Can you work these out from the model? Positions are in its coordinate system, mm. Face numbers are marked on the shaded views. A direction names the side the tool comes from. Give positions to 0.01 mm unless a question says otherwise; leave off trailing zeros. Loops run counter-clockwise (first coordinate to the right, second up) from the corner with the lowest first, then second, coordinate; pieces in that order, holes last.
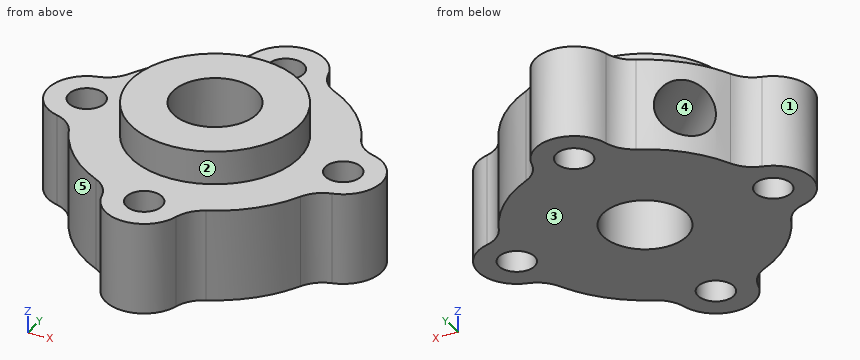
from build123d import *

# Parameters (mm, degrees)
BOSS_EXTRUDE2_DEPTH   = 6.985
FILLET3_R             = 2.54
SKETCH2_R             = 6.35
BOSS_EXTRUDE3_DEPTH   = 2.54
SKETCH3_R             = 3.175
CUT_EXTRUDE1_DEPTH    = 9.525
F_6_32_TAPPED_HOLE1_D = 2.7051
SKETCH12_R            = 2.159
CUT_EXTRUDE4_DEPTH    = 9.906


with BuildPart() as part:
    # Sketch1 → Boss-Extrude2 (new body)
    with BuildSketch(Plane.XY):
        with BuildLine():
            ThreePointArc((-21.795940027, 25.899130336), (-25.822498312, 23.471180796), (-28.250447852, 19.444622511))
            ThreePointArc((-28.250447852, 19.444622511), (-31.607701099, 16.556383583), (-28.250447852, 13.668144655))
            ThreePointArc((-28.250447852, 13.668144655), (-25.822498312, 9.64158637), (-21.795940027, 7.21363683))
            ThreePointArc((-21.795940027, 7.21363683), (-18.907701099, 3.856383583), (-16.019462171, 7.21363683))
            ThreePointArc((-16.019462171, 7.21363683), (-11.992903886, 9.64158637), (-9.564954346, 13.668144655))
            ThreePointArc((-9.564954346, 13.668144655), (-6.207701099, 16.556383583), (-9.564954346, 19.444622511))
            ThreePointArc((-9.564954346, 19.444622511), (-11.992903886, 23.471180796), (-16.019462171, 25.899130336))
            ThreePointArc((-16.019462171, 25.899130336), (-18.907701099, 29.256383583), (-21.795940027, 25.899130336))
        make_face()
    extrude(amount=BOSS_EXTRUDE2_DEPTH)

    # Fillet3
    fillet3_edges = [part.edges().sort_by_distance(p)[0] for p in [
        (-16.019462171, 7.21363683, 3.4925),
        (-21.795940027, 7.21363683, 3.4925),
        (-28.250447852, 13.668144655, 3.4925),
        (-28.250447852, 19.444622511, 3.4925),
        (-21.795940027, 25.899130336, 3.4925),
        (-16.019462171, 25.899130336, 3.4925),
        (-9.564954346, 19.444622511, 3.4925),
        (-9.564954346, 13.668144655, 3.4925),
    ]]
    fillet(fillet3_edges, radius=FILLET3_R)

    # Sketch2 → Boss-Extrude3 (add)
    with BuildSketch(Plane.XY.offset(6.985)):
        with Locations((-18.907701099, 16.556383583)):
            Circle(SKETCH2_R)
    extrude(amount=BOSS_EXTRUDE3_DEPTH)

    # Sketch3 → Cut-Extrude1 (cut)
    with BuildSketch(Plane.XY.offset(9.525)):
        with Locations((-18.907701099, 16.556383583)):
            Circle(SKETCH3_R)
    extrude(amount=-CUT_EXTRUDE1_DEPTH, mode=Mode.SUBTRACT)

    # #6-32 Tapped Hole1 (through all)
    with Locations(Plane(origin=(0, 0, 0), x_dir=(-1, 0, 0), z_dir=(0, 0, -1))):
        with Locations((18.907701099, 26.335383583), (28.686701099, 16.556383583), (18.907701099, 6.777383583), (9.128701099, 16.556383583)):
            Hole(F_6_32_TAPPED_HOLE1_D / 2)

    # Sketch12 → Cut-Extrude4 (cut)
    with BuildSketch(Plane(origin=(-24.434266922, 24.837342139, 0), x_dir=(0.712867541, 0.701298701, 0), z_dir=(-0.701298701, 0.712867541, 0))):
        with Locations((-1.965596828, -3.45963024)):
            Circle(SKETCH12_R)
    extrude(amount=-CUT_EXTRUDE4_DEPTH, mode=Mode.SUBTRACT)


solid = part.part
(1) Please list where these lines run through material, in increasing order: probe 1 along X at (y, z) = (16.5, 9.25); probe 2 along Z at (x, y) = (-24.25, 23) (3 decimals); probe 3 along Z at (x, y) = (-12.75, 10.75) (3 decimals).
Returned:
probe 1: x = -25.26 to -22.08, -15.73 to -12.56
probe 2: z = 0 to 1.458, 5.462 to 6.985
probe 3: z = 0 to 6.985
(2) Will these pins go through, and if not, where does the flat tip stop? P1, Ø3, axis at x = -21.5, z = 6, coming from the -Y side; P2, Ø4, axis at y = 18.5, z = 8.5, coming from the -X side; P3, Ø4.5, axis at x = -18.91, y = 6.78, coming from the +Z side (3 decimals).
Returned:
P1: stops at y = 4.07
P2: stops at x = -31.54
P3: stops at z = 6.985
(3) Which directions (+Z, -Z, +X, -X, +Y, -Y) give clear straight access to the entire face, cutting with the end or side of a thin tool? Please do the marked faces 1 and 2.
Returned:
face 1: +Z, -Z, -X
face 2: +Z
(4) Suppose I cut it at C-C on z = 3. Give the number of separate pieces and of enclosed holes in the cut face, plus the area to 3 significant figures.
Returned:
separate pieces: 1
enclosed holes: 4
area: 277 mm2
(5) Thinking about a two-plate mould opening in Z: for the marked faces 3, 4 and 5, which applies, pulls with the +Z half, pulls with the -Z half, needs draft (parallel to the pull), parting line crosses it, or undercut?
Returned:
face 3: pulls with the -Z half
face 4: undercut
face 5: needs draft
(6) Suppose I cut it at A-A on x = -18.5. List the corners of the cut face in (y, z) for me (3 decimals).
Returned:
outline: (3.885, 0) - (5.488, 0) - (5.488, 6.985) - (3.885, 6.985) - close; (8.067, 0) - (13.408, 0) - (13.408, 9.525) - (10.219, 9.525) - (10.219, 6.985) - (8.067, 6.985) - close; (19.705, 0) - (25.046, 0) - (25.046, 6.985) - (22.893, 6.985) - (22.893, 9.525) - (19.705, 9.525) - close; (27.625, 0) - (29.228, 0) - (29.228, 6.985) - (27.625, 6.985) - close
(7) Suppose I cut it at B-B on y = 14.5. List the corners of the cut face in (x, z) for me (3 decimals).
Returned:
outline: (-30.761, 0) - (-21.327, 0) - (-21.327, 9.525) - (-24.916, 9.525) - (-24.916, 6.985) - (-30.761, 6.985) - close; (-16.489, 0) - (-7.054, 0) - (-7.054, 6.985) - (-12.9, 6.985) - (-12.9, 9.525) - (-16.489, 9.525) - close
